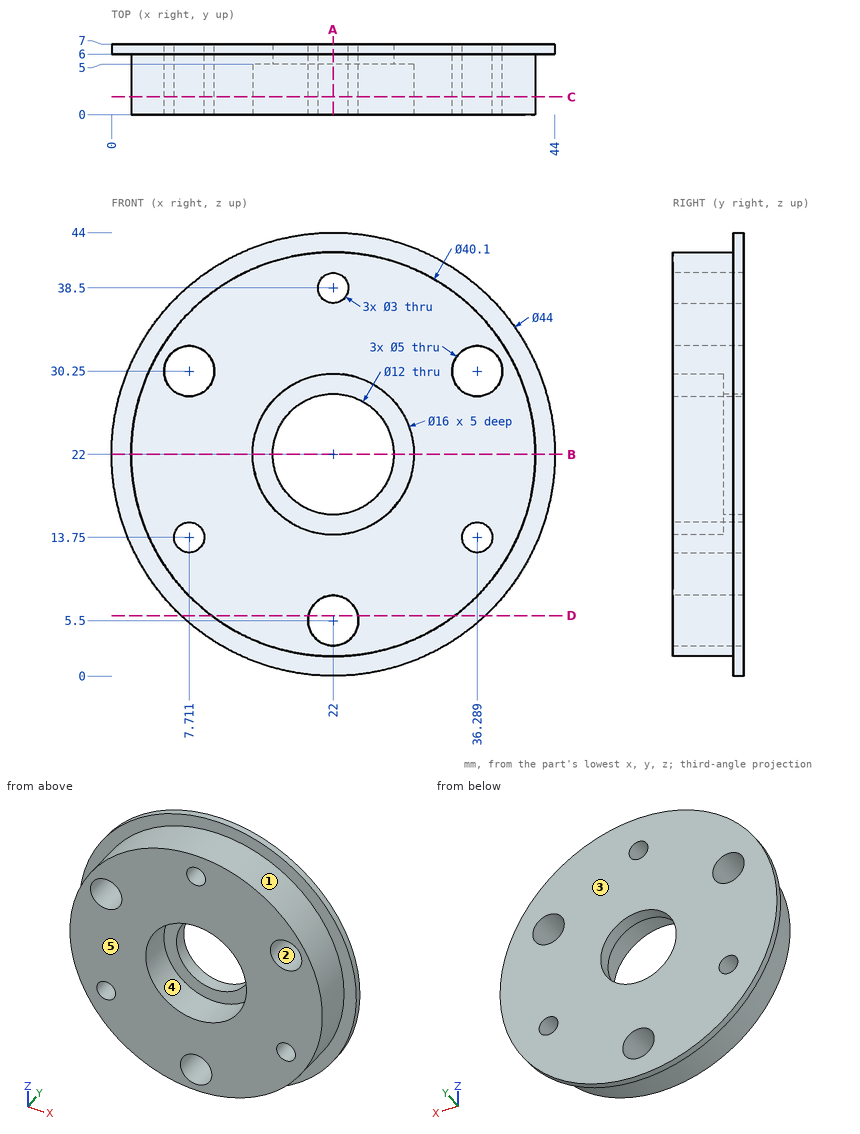
The figure shows three views and two pictorial views of one solid part (mm, origin at its lowest corner). Answer the questions. A direction names the side the tool comes from. Round coordinates to 2 decimals unless told otherwise and drop trailing zeros. Loops run counter-clockwise (first coordinate to the right, second up) from the corner with the lowest first, then second, coordinate; pieces in that order, holes last. Notation, with made-up numbers: M -24,-9.5 L 34,-9.5 A28 ccw 34,17.5 Z; hole C 34,29.25 d6. An arc over 180 degrees is marked long. Return JSON: item names as keys, results as strings.
Q1. Each of these flat-tipped pins is pushed along its axis until it touches: pin 1 Ø1 at (y, z) = (4.5, 11.5) entering from +X; pin 2 Ø1.5 at (y, z) = (5.5, 13.5) entering from +X; pin 3 Ø2 at (x, y) = (23.5, 3.5) entering from -Z. Where does it stop, or does it pass through?
Results list:
{"pin 1": "stops at x = 39.38", "pin 2": "stops at x = 42.52", "pin 3": "stops at z = 1.96"}
Q2. Find the intervals of material crossed by line 1 along X through (y, z) = (5.75, 30.25) (1 decimal); line 2 along Z through (x, y) = (23, 4) (1 decimal); line 3 along X through (y, z) = (2.5, 13.75) (1 decimal), in increasing order. Write a range as from..to.
Results list:
{"line 1": "x = 3.7..5.2, 10.2..33.8, 38.8..40.3", "line 2": "z = 2..3.2, 7.8..14.1, 29.9..37.4, 39.6..42", "line 3": "x = 3.7..6.2, 9.2..34.8, 37.8..40.3"}
Q3. The mould has two halves that part along X. Classify the marked faces 1, 2 and 3: released by +X, released by -X, zero draft, split by the parting line, or undercut.
Results list:
{"face 1": "split by the parting line", "face 2": "undercut", "face 3": "zero draft"}
Q4. Find section A-A, the plane x = 22. Determine the outline of the cut face in (y, z).
Results list:
{"outline": "M 0,1.95 L 6,1.95 L 6,0 L 7,0 L 7,3 L 0,3 Z; M 0,8 L 7,8 L 7,16 L 5,16 L 5,14 L 0,14 Z; M 0,30 L 5,30 L 5,28 L 7,28 L 7,37 L 0,37 Z; M 0,40 L 7,40 L 7,44 L 6,44 L 6,42.05 L 0,42.05 Z"}
Q5. Find section D-D, the plane z = 6. Determine the outline of the cut face in (x, y), plus the area to 3 significant figures.
Results list:
{"outline": "M 6.9,6 L 9.92,6 L 9.92,0 L 19.55,0 L 19.55,7 L 6.9,7 Z; M 24.45,0 L 34.08,0 L 34.08,6 L 37.1,6 L 37.1,7 L 24.45,7 Z", "area": "141 mm2"}
Q6. Find section C-C, the plane y = 1.75. Determine the outline of the cut face in (x, z), plus the area to 3 significant figures.
Results list:
{"outline": "C 22,22 d40.1; hole C 7.71,30.25 d5; hole C 7.71,13.75 d3; hole C 22,22 d16; hole C 22,5.5 d5; hole C 22,38.5 d3; hole C 36.29,30.25 d5; hole C 36.29,13.75 d3", "area": "982 mm2"}
Q7. Find section B-B, the plane z = 22. Determine the outline of the cut face in (x, y).
Results list:
{"outline": "M 0,6 L 1.95,6 L 1.95,0 L 14,0 L 14,5 L 16,5 L 16,7 L 0,7 Z; M 28,5 L 30,5 L 30,0 L 42.05,0 L 42.05,6 L 44,6 L 44,7 L 28,7 Z"}
Q8. Which of the six approach directions +Z, -Z, +X, -X, +Y, -Y give full straight-line access (tool end or side, diameter ignored) to the marked faces 4 and 5?
Results list:
{"face 4": "-Y", "face 5": "+Z, -Z, +X, -X, -Y"}
